from build123d import *

# Parameters (mm, degrees)
SKETCH1_W           = 39.4
SKETCH1_H           = 72.5
BOSS_EXTRUDE1_DEPTH = 3.05
SKETCH4_W           = 1.3
SKETCH4_H           = 0.8
SKETCH4_H_2         = 62
CUT_EXTRUDE1_DEPTH  = 76.190707538
SKETCH7_R           = 1.5
CUT_EXTRUDE4_DEPTH  = 76.190707538


with BuildPart() as part:
    # Sketch1 → Boss-Extrude1 (new body)
    with BuildSketch(Plane(origin=(0, 0, 0), x_dir=(1, 0, 0), z_dir=(0, 1, 0))):
        with Locations((0, 36.25)):
            Rectangle(SKETCH1_W, SKETCH1_H)
    extrude(amount=BOSS_EXTRUDE1_DEPTH)

    # Sketch4 → Cut-Extrude1 (cut, through all)
    with BuildSketch(Plane(origin=(0, 3.05, 0), x_dir=(1, 0, 0), z_dir=(0, 1, 0))):
        with Locations((-0.65, 70.1)):
            Rectangle(SKETCH4_W, SKETCH4_H)
        with Locations((-0.65, 37.5)):
            Rectangle(SKETCH4_W, SKETCH4_H_2)
        with Locations((0.65, 37.5)):
            Rectangle(SKETCH4_W, SKETCH4_H_2)
        with Locations((0.65, 70.1)):
            Rectangle(SKETCH4_W, SKETCH4_H)
    extrude(amount=-CUT_EXTRUDE1_DEPTH, mode=Mode.SUBTRACT)

    # Sketch7 → Cut-Extrude4 (cut, through all)
    with BuildSketch(Plane(origin=(0, 3.05, 0), x_dir=(1, 0, 0), z_dir=(0, 1, 0))):
        with Locations(Location((-12, 5, 0), (0, 0, 270))):
            Circle(SKETCH7_R)
        with Locations(Location((12, 5, 0), (0, 0, 90))):
            Circle(SKETCH7_R)
    extrude(amount=-CUT_EXTRUDE4_DEPTH, mode=Mode.SUBTRACT)


solid = part.part
Read the model definition and answer for the solid it produces. Units are mm, in the model's axes. A direction names the side the tool comes from. Round coordinates to 2 decimals unless told otherwise and drop trailing zeros. Write each loop counter-clockwise with the first axis right and the second up, starting at its lowest first coordinate (ties: lowest second). Pieces come first, ordered by that corner, then holes.
1. Which of the six approach directions +Z, -Z, +X, -X, +Y, -Y give full straight-line access (tool end or side, diameter ignored) to faces 5 (the face through (4, 0, -37)), 6 (the face through (-1.3, 2, -37))?
2. The part is cut by section A-A, the plane z = -5. Determine the outline of the cut face in (x, y).
3. Straight lines are drawn through the part: L1, parallel to X at y = 1.7, z = -5; L2, parallel to X at y = 1.8, z = -52; L3, parallel to Z at x = 12, y = 1.9. For each, find the intervals that lie inside material, in ascending order.
4. Determine the mould class of faces 1 (the face through (0, 2, -72.5)), 2 (the face through (0, 2, -69.7)), 3 (the face through (-19.7, 2, -36)), 4 (the face through (0, 2, 0)) for opening direction Z: pulls with the +Z half, pulls with the -Z half, needs draft (parallel to the pull), parting line crosses it, or undercut.
5. The part is cut by section B-B, the plane x = 0. Determine the outline of the cut face in (y, z).
6. The part is cut by section D-D, the plane x = -12. Determine the outline of the cut face in (y, z).
7. The part is cut by section C-C, the plane y = 2.05. Determine the outline of the cut face in (x, z).
Values:
1. face 5: +Z, -Z, +X, -X, -Y
1. face 6: +Y, -Y
2. outline: (-19.7, 0) - (-13.5, 0) - (-13.5, 3.05) - (-19.7, 3.05) - close; (-10.5, 0) - (10.5, 0) - (10.5, 3.05) - (-10.5, 3.05) - close; (13.5, 0) - (19.7, 0) - (19.7, 3.05) - (13.5, 3.05) - close
3. L1: x = -19.7 to -13.5, -10.5 to 10.5, 13.5 to 19.7
3. L2: x = -19.7 to -1.3, 1.3 to 19.7
3. L3: z = -72.5 to -6.5, -3.5 to 0
4. face 1: pulls with the -Z half
4. face 2: undercut
4. face 3: needs draft
4. face 4: pulls with the +Z half
5. outline: (0, -72.5) - (3.05, -72.5) - (3.05, -70.5) - (0, -70.5) - close; (0, -69.7) - (3.05, -69.7) - (3.05, -68.5) - (0, -68.5) - close; (0, -6.5) - (3.05, -6.5) - (3.05, 0) - (0, 0) - close
6. outline: (0, -72.5) - (3.05, -72.5) - (3.05, -6.5) - (0, -6.5) - close; (0, -3.5) - (3.05, -3.5) - (3.05, 0) - (0, 0) - close
7. outline: (-19.7, -72.5) - (19.7, -72.5) - (19.7, 0) - (-19.7, 0) - close; hole circle Ø3 at (-12, -5); hole (-1.3, -70.5) - (1.3, -70.5) - (1.3, -69.7) - (-1.3, -69.7) - close; hole (-1.3, -68.5) - (1.3, -68.5) - (1.3, -6.5) - (-1.3, -6.5) - close; hole circle Ø3 at (12, -5)
